Can you work these out from the model? Positions are in its coordinate system, mm. Face numbers are marked on the shaded views. A direction names the side the tool comes from. Give positions to 0.01 mm unless a question says otherwise; leave off trailing zeros. Order: outer loops, then holes, each group sorted by start corner. A loop starts at its lowest first (then second) coordinate and runs counter-clockwise, first axis right, second up.
Item 1: I want a section at C-C, the plane x = 15. Write out the boundary of the cut face in (y, z), then the cut area to 3 significant figures.
Item 2: I want a section at B-B, the plane z = 79. Write out the boundary of the cut face in (x, y), then the cut area to 3 significant figures.
Item 3: If I drill on line 1 along Z through (x, y) = (67, -3.55); line 2 along Z through (x, y) = (46, -1.5); line 3 along Z through (x, y) = (68, -0.75), over which ranges is the centre line in solid material (lowest first)?
Item 4: I want a section at A-A, the plane x = 149.5. Write out the boundary of the cut face in (y, z), then the cut area to 3 significant figures.
Item 5: I want a section at D-D, the plane z = 46. Write out the boundary of the cut face in (x, y).
Item 6: Which directions (+Z, -Z, +X, -X, +Y, -Y) give clear straight access to the entire face, cutting with the end or side of a thin tool? Please do the marked faces 1 and 2.
Item 7: I'm going to push flat-ended pins straight in: pin 1 Ø1.5 at (x, y) = (130.5, 3.5) entering from +Z; pin 2 Ø2 at (y, z) = (2.5, 7) entering from +X; pin 3 Ø1.5 at (x, y) = (19, -1.5) entering from +Z. Where does each tip first touch, or does it pass through?
```python
from build123d import *

# Parameters (mm, degrees)
SKETCH_R     = 5
PAD_DEPTH    = 8
PAD001_DEPTH = 13
FILLET_R     = 3
FILLET001_R  = 5
FILLET002_R  = 20
FILLET003_R  = 5
FILLET004_R  = 3


with BuildPart() as part:
    # Sketch → Pad (new body)
    with BuildSketch(Plane.XZ):
        Polygon((0, 0), (66, 0), (66, 40), (176, 40), (176, 90), (51, 90), (51, 70), (11, 70), (0, 70), align=None)
        with Locations((67, 65)):
            Circle(SKETCH_R, mode=Mode.SUBTRACT)
    extrude(amount=PAD_DEPTH)

    # Sketch001 (on Face12 of Pad) → Pad001 (join)
    with BuildSketch(Plane.XZ.offset(8)):
        Polygon((66, 0), (66, 40), (176, 40), (176, 32), (74, 32), (74, 0), align=None)
    extrude(amount=-PAD001_DEPTH)

    # Fillet
    fillet_edges = [part.edges().sort_by_distance(p)[0] for p in [
        (176, -4, 90),
        (51, -4, 90),
        (51, -4, 70),
        (0, -4, 70),
    ]]
    fillet(fillet_edges, radius=FILLET_R)

    # Fillet001
    fillet001_edges = [part.edges().sort_by_distance(p)[0] for p in [
        (0, -8, 33.5),
    ]]
    fillet(fillet001_edges, radius=FILLET001_R)

    # Fillet002
    fillet002_edges = [part.edges().sort_by_distance(p)[0] for p in [
        (66, 2.5, 40),
        (74, -1.5, 32),
    ]]
    fillet(fillet002_edges, radius=FILLET002_R)

    # Fillet003
    fillet003_edges = [part.edges().sort_by_distance(p)[0] for p in [
        (79.857864, -8, 26.142136),
        (74, -1.5, 0),
    ]]
    fillet(fillet003_edges, radius=FILLET003_R)

    # Fillet004
    fillet004_edges = [part.edges().sort_by_distance(p)[0] for p in [
        (62, -8, 65),
        (62, 0, 65),
    ]]
    fillet(fillet004_edges, radius=FILLET004_R)


solid = part.part
```
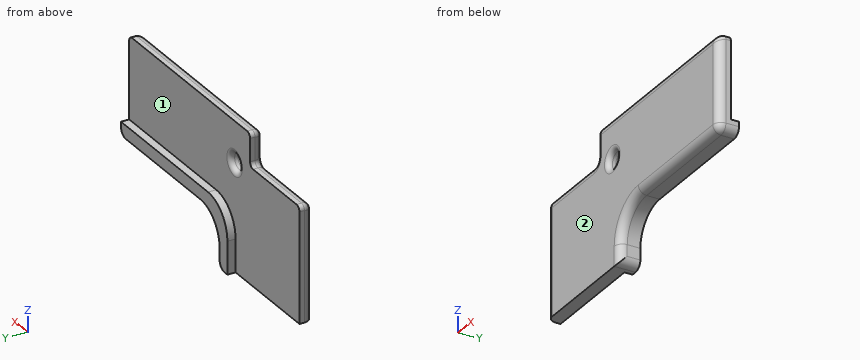
Results list:
1. outline: (-8, 0) - (0, 0) - (0, 70) - (-3, 70) arc R5 ccw to (-8, 65) - close
1. area: 555 mm2
2. outline: (51, -3) arc R5 ccw to (56, -8) - (171, -8) arc R5 ccw to (176, -3) - (176, 0) - (51, 0) - close
2. area: 989 mm2
3. line 1: z = 0 to 60, 70 to 89.97
3. line 2: z = 0 to 70
3. line 3: z = 0 to 59.07, 70.93 to 90
4. outline: (-8, 37) arc R5 ccw to (-3, 32) - (5, 32) - (5, 40) - (0, 40) - (0, 90) - (-3, 90) arc R5 ccw to (-8, 85) - close
4. area: 493 mm2
5. outline: (0, -3) arc R5 ccw to (5, -8) - (171, -8) arc R5 ccw to (176, -3) - (176, 0) - (0, 0) - close
6. face 1: +Z, -X, +Y
6. face 2: +Z, -Z, +X, -X, -Y
7. pin 1: stops at z = 40
7. pin 2: stops at x = 74
7. pin 3: stops at z = 70
